Can you work these out from the model? Positions are in its coordinate system, mm. A direction names the side the tool comes from. Coordinates: 2 decimals unless noted, no trailing zeros. Loops run counter-clockwise (first coordinate to the right, second up) from the corner with the lowest first, then second, coordinate; pieces in that order, holes last.
```python
from build123d import *

# Parameters (mm, degrees)
F0_W      = 31.61
F0_H      = 15.57
F1_DEPTH  = 15.71
F2_W      = 7.63
F2_H      = 15.77
F3_DEPTH  = 15.55
F5_DEPTH  = 7.97
F7_DEPTH  = 25
F8_W      = 7.1303485631
F8_H      = 8.063195222
F9_DEPTH  = 25
F10_SIZE2 = 7.6
F10_SIZE  = 8.4


with BuildPart() as f1:
    # F0 (on Top) → F1 (new body)
    with BuildSketch(Plane.XY):
        with Locations((-0.5104932934, 0.6546514369)):
            Rectangle(F0_W, F0_H)
    extrude(amount=F1_DEPTH)

    # F2 (on face) → F3 (join)
    with BuildSketch(Plane.XZ.offset(7.1303485631)):
        with Locations((11.4795067066, 23.595)):
            Rectangle(F2_W, F2_H)
    extrude(amount=-F3_DEPTH)

    # F4 (on face) → F5 (cut)
    with BuildSketch(Plane.XZ.offset(7.1303485631)):
        Polygon((-0.4054932934, 0), (-0.4054932934, 8.01), (-8.0654932934, 8.01), (-16.3154932934, 8.01), (-16.3154932934, 0), align=None)
    extrude(amount=-F5_DEPTH, mode=Mode.SUBTRACT)

    # F6 (on face) → F7 (cut)
    with BuildSketch(Plane.XY.offset(15.71)):
        Polygon((0, 0), (-7.9760523513, -7.1303485631), (0, -7.1303485631), align=None)
    extrude(amount=-F7_DEPTH, mode=Mode.SUBTRACT)

    # F8 (on face) → F9 (cut)
    with BuildSketch(Plane.YZ.offset(15.2945067066)):
        with Locations((-3.5651742816, 19.741597611)):
            Rectangle(F8_W, F8_H)
    extrude(amount=-F9_DEPTH, mode=Mode.SUBTRACT)

    # F10
    f10_edges = [f1.edges().sort_by_distance(p)[0] for p in [
        (7.664507, 0, 19.741598),
    ]]
    f10_side = f1.faces().sort_by_distance((7.664507, 1.933934, 24.775126))[0]
    chamfer(f10_edges, length=F10_SIZE, length2=F10_SIZE2, reference=f10_side)


solid = f1.part
```
Item 1: We'd pull the mould along X, two halves only. Please class faces 1 (the face through (-3.932, -3.515, 11.456)), 2 (the face through (11, 8.42, 24)), 3 (the face through (15.295, 1, 16)): +X half, -X half, draft (parallel to the pull), parting line (faces both ways), or undercut.
Results are:
face 1: undercut
face 2: draft
face 3: +X half
Item 2: Suppose I cut it at B-B, the plane y = -2.5. Please give me the cut outline in (x, z).
Results are:
outline: (-16.32, 8.01) - (-2.8, 8.01) - (-2.8, 15.71) - (-16.32, 15.71) - close; (0, 0) - (15.29, 0) - (15.29, 15.71) - (0, 15.71) - close; (7.66, 23.77) - (15.29, 23.77) - (15.29, 31.48) - (7.66, 31.48) - close
Item 3: I need wall thicknesses on line 1 along Z through (x, y) = (14.5, -1.5); line 2 along Z through (x, y) = (-11, -2); line 3 along Z through (x, y) = (-1, 2). Which ranges of each line are inside material? Lowest first, please.
Results are:
line 1: z = 0 to 15.71, 23.77 to 31.48
line 2: z = 8.01 to 15.71
line 3: z = 0 to 15.71
Item 4: On a 3-axis mill with a long thin cutter (end or side, diameter ignored), from which of +Z, -Z, +X, -X, +Y, -Y can I reach the whole of each face in a straight line? I mean faces 4 (the face through (-16.315, 2, 9)), 5 (the face through (11, -1, 23.773)), 6 (the face through (7.665, 1, 27)), 7 (the face through (0, -4, 8)), 8 (the face through (-8, 0.84, 4)). Say none if no direction works.
Results are:
face 4: +Z, -Z, -X, +Y, -Y
face 5: -X, -Y
face 6: +Z, -X, +Y, -Y
face 7: +Z, -Z, -Y
face 8: -Z, -X, -Y
Item 5: I'm going to push flat-ended pins straight in: P1, Ø0.6, axis at y = 0.5, z = 2.5, coming from the -X side; P2, Ø6, axis at x = 2, y = 0, coming from the +Z side; P3, Ø4, axis at x = 12, z = 26.5, coming from the +Y side. Where does each tip first touch, or does it pass through?
Results are:
P1: stops at x = -0.41
P2: stops at z = 15.71
P3: stops at y = 8.42
Item 6: Suppose I cut it at D-D, the plane z = 2. Please give me the cut outline in (x, y).
Results are:
outline: (-16.32, 0.84) - (-0.41, 0.84) - (-0.41, -0.36) - (0, 0) - (0, -7.13) - (15.29, -7.13) - (15.29, 8.44) - (-16.32, 8.44) - close
